CAD build for the part. Positions are in the model's coordinates, mm. Give positions to 0.01 mm unless a question says otherwise; leave off trailing zeros. Loops run counter-clockwise (first coordinate to the right, second up) from the corner with the lowest first, then second, coordinate; pieces in that order, holes last.
```python
from build123d import *

# Parameters (mm, degrees)
F4_R     = 3.175
F5_DEPTH = 25.4


with BuildPart() as f2:
    # F1 (on Top) → F2 (revolve)
    with BuildSketch(Plane.XY):
        with BuildLine():
            Line((0, -15.875), (0, 15.875))
            ThreePointArc((0, 15.875), (-15.875, 0), (0, -15.875))
        make_face()
    revolve(axis=Axis((0, 0, 0), (0, -1, 0)))


with BuildPart() as f5:
    # F4 (on offset) → F5 (new body)
    with BuildSketch(Plane.XZ.offset(6.35)):
        Circle(F4_R)
    extrude(amount=F5_DEPTH)


with BuildPart() as f2_1:
    add(f2.part)

    # F6: cut F5
    add(f5.part, mode=Mode.SUBTRACT)


solid = f2_1.part
```
1. Saw through at B-B, the plane z = 0. List the corners of the cut face in (x, y) (3 decimals).
Responses:
outline: (-3.175, -15.554) - (-3.175, -6.35) - (3.175, -6.35) - (3.175, -15.554) arc R15.875 ccw (long way) to start
2. Pull direction Z, two halves, no side cores. Call faces 1 (the face through (0, -6.35, 0)), 2 (the face through (-0.69, -10.89, -3.1)): released by +Z, released by -Z, zero draft, split by the parting line, or undercut.
Responses:
face 1: undercut
face 2: undercut
3. Drop flat-ended pins along their axis: pin 1 (1.9 mm diameter, centred on x = -1, z = -1, fed in from -Y); pin 2 (12 mm diameter, centred on x = -0.5, z = -8.5, fed in from +Y); pin 3 (12 mm diameter, centred on x = -7.5, z = -11.5, fed in from +Y). Give the stop position or say it passes through.
Responses:
pin 1: stops at y = -6.35
pin 2: stops at y = 15.67
pin 3: stops at y = 13.87
4. Probe line 1 along Z through (x, y) = (0, -9.5) (3 decimals); line 2 along Z through (x, y) = (0, -13.25) (3 decimals); line 3 along X through (y, z) = (-10.5, 0) (3 decimals). List the from-to ranges inside material, lowest first.
Responses:
line 1: z = -12.719 to -3.175, 3.175 to 12.719
line 2: z = -8.744 to -3.175, 3.175 to 8.744
line 3: x = -11.907 to -3.175, 3.175 to 11.907
5. Saw through at D-D, the plane y = -1.5. List the corners of the cut face in (x, z), and give its area (3 significant figures).
Responses:
outline: circle Ø31.61 at (0, 0)
area: 785 mm2
6. Saw through at C-C, the plane y = -9. List the corners of the cut face in (x, z) (3 decimals), and give its area (3 significant figures).
Responses:
outline: circle Ø26.155 at (0, 0); hole circle Ø6.35 at (0, 0)
area: 506 mm2
7. Saw through at A-A, the plane x = 0. List the corners of the cut face in (y, z) (3 decimals), and give its area (3 significant figures).
Responses:
outline: (-15.554, -3.175) arc R15.875 ccw (long way) to (-15.554, 3.175) - (-6.35, 3.175) - (-6.35, -3.175) - close
area: 732 mm2
